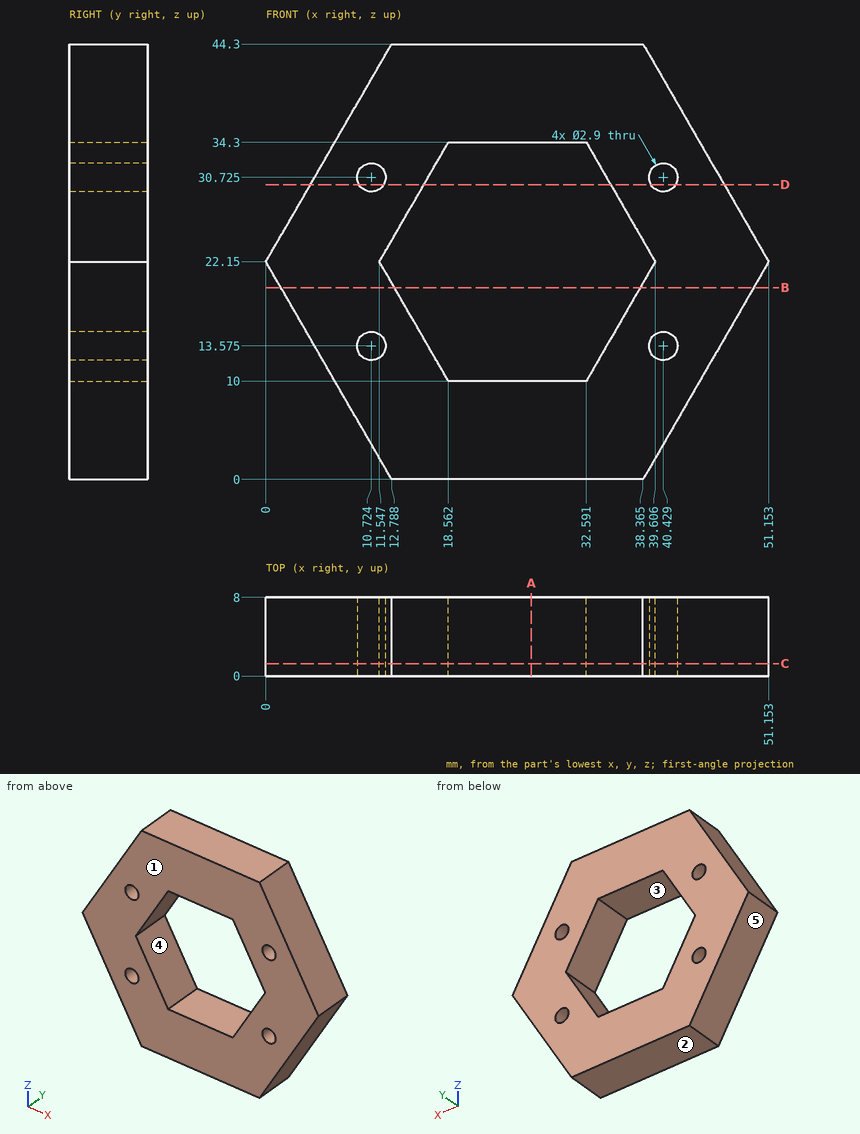
Part print with two shaded views. Sizes in mm from the minimum x, y, z corner. A direction names the side the tool comes from. Round coordinates to 2 decimals unless told otherwise and drop trailing zeros. Write each loop counter-clockwise with the first axis right and the second up, starting at its lowest first coordinate (ties: lowest second). Pieces come first, ordered by that corner, then holes. Notation, with made-up numbers: M 44,-16 L 93,-16 A12 ccw 93,0 Z; hole C -2,-14.5 d5. An arc over 180 degrees is marked long. Answer as CSV lines item,"result". Start each with the question number.
1) Drill centre lines: L1, parallel to Z at x = 31, y = 5.25; L2, parallel to Z at x = 40.5, y = 2.75 (1 decimal); L3, parallel to Z at x = 40, y = 7.25 (1 decimal). Where is each one in solid material? Low to high.
2) Band-saw the part on C-C (y = 1.25). Count the separate pieces of the cut face and the enclosed holes in it, then the cut area to 3 significant figures.
3) Band-saw the part on D-D (z = 30). List the corners of the cut face in (x, y) (1 decimal).
4) Mould opens along Z. For the marked faces 1, 2 and 3 say: +Z half, -Z half, draft (parallel to the pull), parting line (faces both ways), or undercut.
5) Drop flat-ended pins along their axis: pin 1 (1 mm diameter, centred on y = 3, z = 33.5, fed in from +X); pin 2 (4 mm diameter, centred on y = 6, z = 11.5, fed in from -X) (1 decimal); pin 3 (3 mm diameter, centred on x = 42.5, y = 3.5, fed in from +Z) (1 decimal). Give the stop position or say it passes through.
6) Band-saw the part on A-A (x = 27). List the corners of the cut face in (y, z), then the cut area to 3 significant figures.
7) Which spindle directions (+Z, -Z, +X, -X, +Y, -Y) get a long thin tool onto all of the face, cutting with end or side? Do the marked faces 4 and 5. Say none if no direction does.
8) Band-saw the part on B-B (z = 19.5). List the corners of the cut face in (x, y).
Worked out:
1,L1,"0 to 10, 34.3 to 44.3"
1,L2,"3.7 to 12.1, 15 to 29.3, 32.2 to 40.6"
1,L3,"2.8 to 12.2, 15 to 29.3, 32.1 to 41.5"
2,separate pieces,"1"
2,enclosed holes,"5"
2,area,"1,160 mm²"
3,outline,"M 4.5,0 L 9.5,0 L 9.5,8 L 4.5,8 Z; M 12,0 L 16.1,0 L 16.1,8 L 12,8 Z; M 35.1,0 L 39.2,0 L 39.2,8 L 35.1,8 Z; M 41.7,0 L 46.6,0 L 46.6,8 L 41.7,8 Z"
4,face 1,"draft"
4,face 2,"-Z half"
4,face 3,"undercut"
5,pin 1,"x = 44.89"
5,pin 2,"x = 5"
5,pin 3,"z = 39.7"
6,outline,"M 0,0 L 8,0 L 8,10 L 0,10 Z; M 0,34.3 L 8,34.3 L 8,44.3 L 0,44.3 Z"
6,area,"160 mm²"
7,face 4,"+Y, -Y"
7,face 5,"-Z, -X, +Y, -Y"
8,outline,"M 1.53,0 L 13.08,0 L 13.08,8 L 1.53,8 Z; M 38.08,0 L 49.62,0 L 49.62,8 L 38.08,8 Z"
